```python
from build123d import *

# Parameters (mm, degrees)
F0_W     = 30.5
F0_H     = 30.5
F1_DEPTH = 30
F2_R     = 25.75
F2_W     = 30.5
F2_H     = 30.5
F2_R_2   = 15
F3_DEPTH = 1
F4_R     = 25.75
F4_R_2   = 15.4
F5_DEPTH = 30.5


# Not quite as in the source:
# - a feature names something its author has since deleted; it is built from what else it names


with BuildPart() as f1:
    # F0 (on Top) → F1 (new body)
    with BuildSketch(Plane.XY):
        Rectangle(F0_W, F0_H)
    extrude(amount=F1_DEPTH)

    # F2 (on face) → F3 (join)
    with BuildSketch(Plane(origin=(0, 0, 0), x_dir=(1, 0, 0), z_dir=(0, 0, -1))):
        Circle(F2_R)
        Rectangle(F2_W, F2_H, mode=Mode.SUBTRACT)
        Rectangle(F2_W, F2_H)
        Circle(F2_R_2, mode=Mode.SUBTRACT)
        Circle(F2_R_2)
    extrude(amount=F3_DEPTH)

    # F4 (on face) → F5 (join)
    with BuildSketch(Plane(origin=(0, 0, -1), x_dir=(1, 0, 0), z_dir=(0, 0, -1))):
        Circle(F4_R)
        Circle(F4_R_2, mode=Mode.SUBTRACT)
    extrude(amount=F5_DEPTH)


solid = f1.part
```
Can you work these out from the model? Positions are in its coordinate system, mm. A direction names the side the tool comes from. Coordinates: 2 decimals unless noted, no trailing zeros. Loops run counter-clockwise (first coordinate to the right, second up) from the corner with the lowest first, then second, coordinate; pieces in that order, holes last.
Item 1: I'm going to push flat-ended pins straight in: pin 1 (1 mm diameter, centred on x = -10, z = -15.5, fed in from -Y); pin 2 (1 mm diameter, centred on x = 4.5, z = 15.5, fed in from +Y); pin 3 (3 mm diameter, centred on x = -19, z = -1, fed in from +Y); pin 4 (6 mm diameter, centred on x = -20, z = 23, fed in from -Y). Where does each tip first touch, or does it pass through?
Answers below:
pin 1: stops at y = -23.93
pin 2: stops at y = 15.25
pin 3: stops at y = 18.89
pin 4: passes through
Item 2: Please list where these lines run through material, in increasing order: L1, parallel to X at y = 0, z = -16; L2, parallel to Y at x = 15, z = 6.
Answers below:
L1: x = -25.75 to -15.4, 15.4 to 25.75
L2: y = -15.25 to 15.25
Item 3: Suppose I cut it at C-C (z = -18). Please give me the cut outline in (x, y).
Answers below:
outline: circle Ø51.5 at (0, 0); hole circle Ø30.8 at (0, 0)
Item 4: Which directions (+Z, -Z, +X, -X, +Y, -Y) give clear straight access to the entire face, cutting with the end or side of a thin tool? Please do faces 5 (the face through (0, 0, 30)), 6 (the face through (0, 0, -1)), 7 (the face through (15.25, 0, 15)), 8 (the face through (0, 15.25, 15)).
Answers below:
face 5: +Z, +X, -X, +Y, -Y
face 6: -Z
face 7: +Z, +X, +Y, -Y
face 8: +Z, +X, -X, +Y
Item 5: Suppose I cut it at D-D (z = 3). Please give me the cut outline in (x, y).
Answers below:
outline: (-15.25, -15.25) - (15.25, -15.25) - (15.25, 15.25) - (-15.25, 15.25) - close
Item 6: Suppose I cut it at A-A (x = 0). Please give me the cut outline in (y, z).
Answers below:
outline: (-25.75, -31.5) - (-15.4, -31.5) - (-15.4, -1) - (15.4, -1) - (15.4, -31.5) - (25.75, -31.5) - (25.75, 0) - (15.25, 0) - (15.25, 30) - (-15.25, 30) - (-15.25, 0) - (-25.75, 0) - close
Item 7: If we mould it in two halves opening along X, with no side actions, what happens to faces 1 (the face through (-3.338, 15.034, -16.036)), 2 (the face through (0, -15.25, 15)), 3 (the face through (-5.58, 25.14, -15.53)), 4 (the face through (-15.25, 0, 15))? For each: released by +X, released by -X, zero draft, split by the parting line, or undercut.
Answers below:
face 1: undercut
face 2: zero draft
face 3: split by the parting line
face 4: released by -X
